```python
from build123d import *

# Parameters (mm, degrees)
SKETCH_1_W                = 100
SKETCH_1_H                = 130
EXTRUDE_1_DEPTH           = 3
SKETCH_2_R                = 2.1
CUT_EXTRUDE_1_DEPTH       = 83.060952956
SKETCH_5_W                = 100
SKETCH_5_H                = 130
EXTRUDE_2_DEPTH           = 3
CUT_EXTRUDE_4_DEPTH       = 164.505351594
CUT_EXTRUDE_4_DEPTH_BACK  = 164.505351594
SKETCH_6_R                = 2.1
CUT_EXTRUDE_5_DEPTH       = 164.505351594
CUT_EXTRUDE_5_DEPTH_BACK  = 164.505351594
SKETCH_7_R                = 2.55
CUT_EXTRUDE_6_DEPTH       = 164.505351594
CUT_EXTRUDE_6_DEPTH_BACK  = 164.505351594
CUT_EXTRUDE_7_DEPTH       = 164.505351594
CUT_EXTRUDE_7_DEPTH_BACK  = 164.505351594
SKETCH_12_W               = 20
SKETCH_12_H               = 20
CUT_EXTRUDE_8_DEPTH       = 164.505351594
CUT_EXTRUDE_8_DEPTH_BACK  = 164.505351594
SKETCH_13_W               = 200
SKETCH_13_H               = 20
CUT_EXTRUDE_9_DEPTH       = 164.505351594
CUT_EXTRUDE_9_DEPTH_BACK  = 164.505351594
SKETCH_14_W               = 5
SKETCH_14_H               = 90
CUT_EXTRUDE_10_DEPTH      = 159.930802553
CUT_EXTRUDE_10_DEPTH_BACK = 159.930802553
SKETCH_15_R               = 1.25
SKETCH_15_R_2             = 22
CUT_EXTRUDE_11_DEPTH      = 159.930802553
CUT_EXTRUDE_11_DEPTH_BACK = 159.930802553
FILLET_1_R                = 1


with BuildPart() as part:
    # 草图1 → 凸台-拉伸1 (new body)
    with BuildSketch(Plane.XY):
        Rectangle(SKETCH_1_W, SKETCH_1_H)
    extrude(amount=EXTRUDE_1_DEPTH)

    # 草图2 → 切除-拉伸1 (cut, through all)
    with BuildSketch(Plane.XY.offset(3)):
        with Locations((-40, 55)):
            Circle(SKETCH_2_R)
        with Locations((-20, 55)):
            Circle(SKETCH_2_R)
        with Locations((0, 55)):
            Circle(SKETCH_2_R)
        with Locations((20, 55)):
            Circle(SKETCH_2_R)
        with Locations((40, 55)):
            Circle(SKETCH_2_R)
        with Locations((-40, -55)):
            Circle(SKETCH_2_R)
        with Locations(Location((40, -55, 0), (0, 0, 180))):
            Circle(SKETCH_2_R)
        with Locations(Location((20, -55, 0), (0, 0, 180))):
            Circle(SKETCH_2_R)
        with Locations(Location((0, -55, 0), (0, 0, 180))):
            Circle(SKETCH_2_R)
        with Locations(Location((-20, -55, 0), (0, 0, 180))):
            Circle(SKETCH_2_R)
    extrude(amount=-CUT_EXTRUDE_1_DEPTH, mode=Mode.SUBTRACT)

    # 草图5 → 凸台-拉伸2 (add)
    with BuildSketch(Plane.XY.offset(3)):
        with Locations((100, 0)):
            Rectangle(SKETCH_5_W, SKETCH_5_H)
    extrude(amount=-EXTRUDE_2_DEPTH)

    # 草图6 → 切除-拉伸4 (cut, two sides: drawn at the far end of the back side and taken through both)
    with BuildSketch(Plane.XY.offset(3).offset(-CUT_EXTRUDE_4_DEPTH_BACK)):
        with Locations((55, 55)):
            Circle(SKETCH_6_R)
        with Locations((70, 55)):
            Circle(SKETCH_6_R)
        with Locations((85, 55)):
            Circle(SKETCH_6_R)
        with Locations((100, 55)):
            Circle(SKETCH_6_R)
        with Locations((115, 55)):
            Circle(SKETCH_6_R)
        with Locations((130, 55)):
            Circle(SKETCH_6_R)
        with Locations((145, 55)):
            Circle(SKETCH_6_R)
        with Locations((145, -55)):
            Circle(SKETCH_6_R)
        with Locations((130, -55)):
            Circle(SKETCH_6_R)
        with Locations((115, -55)):
            Circle(SKETCH_6_R)
        with Locations((100, -55)):
            Circle(SKETCH_6_R)
        with Locations((85, -55)):
            Circle(SKETCH_6_R)
        with Locations((70, -55)):
            Circle(SKETCH_6_R)
        with Locations((55, -55)):
            Circle(SKETCH_6_R)
    extrude(amount=CUT_EXTRUDE_4_DEPTH + CUT_EXTRUDE_4_DEPTH_BACK, mode=Mode.SUBTRACT)

    # 草图7 → 切除-拉伸5 (cut, two sides: drawn at the far end of the back side and taken through both)
    with BuildSketch(Plane(origin=(0, 0, 0), x_dir=(-1, 0, 0), z_dir=(0, 0, -1)).offset(-CUT_EXTRUDE_5_DEPTH_BACK)):
        with Locations((-140, -30)):
            Circle(SKETCH_7_R)
        with Locations((-120, -30)):
            Circle(SKETCH_7_R)
        with Locations((-100, -30)):
            Circle(SKETCH_7_R)
        with Locations((-80, -30)):
            Circle(SKETCH_7_R)
        with Locations((-60, -30)):
            Circle(SKETCH_7_R)
        with Locations((-40, -30)):
            Circle(SKETCH_7_R)
        with Locations((-20, -30)):
            Circle(SKETCH_7_R)
        with Locations((0, -30)):
            Circle(SKETCH_7_R)
        with Locations((20, -30)):
            Circle(SKETCH_7_R)
        with Locations((40, -30)):
            Circle(SKETCH_7_R)
    extrude(amount=CUT_EXTRUDE_5_DEPTH + CUT_EXTRUDE_5_DEPTH_BACK, mode=Mode.SUBTRACT)

    # 草图11 → 切除-拉伸6 (cut, two sides: drawn at the far end of the back side and taken through both)
    with BuildSketch(Plane.XY.offset(3).offset(-CUT_EXTRUDE_6_DEPTH_BACK)):
        with BuildLine():
            Line((74.5, 19.5), (74.5, 65))
            Line((74.5, 65), (25.5, 65))
            Line((25.5, 65), (25.5, 19.5))
            ThreePointArc((25.5, 19.5), (50, -5), (74.5, 19.5))
        make_face()
    extrude(amount=CUT_EXTRUDE_6_DEPTH + CUT_EXTRUDE_6_DEPTH_BACK, mode=Mode.SUBTRACT)

    # 草图12 → 切除-拉伸7 (cut, two sides: drawn at the far end of the back side and taken through both)
    with BuildSketch(Plane.XY.offset(3).offset(-CUT_EXTRUDE_7_DEPTH_BACK)):
        with Locations((-40, 55)):
            Rectangle(SKETCH_12_W, SKETCH_12_H)
        with Locations((140, 55)):
            Rectangle(SKETCH_12_W, SKETCH_12_H)
    extrude(amount=CUT_EXTRUDE_7_DEPTH + CUT_EXTRUDE_7_DEPTH_BACK, mode=Mode.SUBTRACT)

    # 草图13 → 切除-拉伸8 (cut, two sides: drawn at the far end of the back side and taken through both)
    with BuildSketch(Plane.XY.offset(3).offset(-CUT_EXTRUDE_8_DEPTH_BACK)):
        with Locations((50, -55)):
            Rectangle(SKETCH_13_W, SKETCH_13_H)
    extrude(amount=CUT_EXTRUDE_8_DEPTH + CUT_EXTRUDE_8_DEPTH_BACK, mode=Mode.SUBTRACT)

    # 草图14 → 切除-拉伸9 (cut, two sides: drawn at the far end of the back side and taken through both)
    with BuildSketch(Plane.XY.offset(3).offset(-CUT_EXTRUDE_9_DEPTH_BACK)):
        with Locations((147.5, 0)):
            Rectangle(SKETCH_14_W, SKETCH_14_H)
    extrude(amount=CUT_EXTRUDE_9_DEPTH + CUT_EXTRUDE_9_DEPTH_BACK, mode=Mode.SUBTRACT)

    # 草图15 → 切除-拉伸10 (cut, two sides: drawn at the far end of the back side and taken through both)
    with BuildSketch(Plane(origin=(0, 0, 0), x_dir=(-1, 0, 0), z_dir=(0, 0, -1)).offset(-CUT_EXTRUDE_10_DEPTH_BACK)):
        with Locations((10.74, 4.505)):
            Circle(SKETCH_15_R)
        with Locations((31.96195252, -32.2525)):
            Circle(SKETCH_15_R)
        with Locations((-10.48195252, -32.2525)):
            Circle(SKETCH_15_R)
        with Locations((10.74, -20)):
            Circle(SKETCH_15_R_2)
    extrude(amount=CUT_EXTRUDE_10_DEPTH + CUT_EXTRUDE_10_DEPTH_BACK, mode=Mode.SUBTRACT)

    # 草图16 → 切除-拉伸11 (cut, two sides: drawn at the far end of the back side and taken through both)
    with BuildSketch(Plane.XY.offset(3).offset(-CUT_EXTRUDE_11_DEPTH_BACK)):
        Polygon((6, 10.5), (6, 28.5), (25.5, 28.5), (74.5, 28.5), (123, 28.5), (123, 10.5), (74.5, 10.5), (25.5, 10.5), align=None)
    extrude(amount=CUT_EXTRUDE_11_DEPTH + CUT_EXTRUDE_11_DEPTH_BACK, mode=Mode.SUBTRACT)

    # 圆角1
    fillet_1_edges = [part.edges().sort_by_distance(p)[0] for p in [
        (74.5, 28.5, 1.5),
        (27.21294227, 10.5, 1.5),
        (72.78705773, 10.5, 1.5),
        (123, 10.5, 1.5),
        (25.5, 28.5, 1.5),
        (6, 28.5, 1.5),
        (6, 10.5, 1.5),
        (123, 28.5, 1.5),
    ]]
    fillet(fillet_1_edges, radius=FILLET_1_R)


solid = part.part
```
Here's how the part is built. I have some questions about the finished solid (model axes, mm). Coordinates: 2 decimals unless noted, no trailing zeros. Loops run counter-clockwise (first coordinate to the right, second up) from the corner with the lowest first, then second, coordinate; pieces in that order, holes last. Notation, with made-up numbers: M 79.25,56 L 122.25,56 A3 cw 122.25,60 Z; hole C 10.25,33.5 d4. An arc over 180 degrees is marked long. One line per item, written item: value.
1. Will these pins go through, and if not, where does the flat tip stop? pin 1 Ø1.5 at (y, z) = (62, 1) entering from +X; pin 2 Ø4 at (x, y) = (100, 55) entering from -Z; pin 3 Ø1.5 at (x, z) = (137.5, 1.5) entering from +Y; pin 4 Ø6.5 at (x, y) = (40, -30) entering from -Z.
Geometry says:
pin 1: stops at x = 130
pin 2: passes through
pin 3: stops at y = 45
pin 4: stops at z = 0
2. Please list where these lines run through material, in increasing order: probe 1 along Y at (x, z) = (20, 1.8); probe 2 along Y at (x, z) = (85.5, 1.6); probe 3 along X at (y, z) = (22.5, 2.85).
Geometry says:
probe 1: y = -45 to -32.55, -27.45 to 10.5, 28.5 to 52.9, 57.1 to 65
probe 2: y = -45 to 10.5, 28.5 to 52.96, 57.04 to 65
probe 3: x = -50 to 6, 123 to 145
3. Thinking about a two-plate mould opening in X: for faces 1 (the cylindrical face through (50, -5, 1)), 2 (the flat face through (46, -14, 0)), 3 (the cylindrical face through (62.548, -29.888, 1.521)), which applies, +X half, -X half, draft (parallel to the pull), parting line (faces both ways), or undercut?
Geometry says:
face 1: undercut
face 2: draft
face 3: undercut
4. Imagine slicing it at A-A (x = 100). List the corners of the cut face in (y, z) for me, and give its area (3 significant figures).
Geometry says:
outline: M -45,0 L -32.55,0 L -32.55,3 L -45,3 Z; M -27.45,0 L 10.5,0 L 10.5,3 L -27.45,3 Z; M 28.5,0 L 52.9,0 L 52.9,3 L 28.5,3 Z; M 57.1,0 L 65,0 L 65,3 L 57.1,3 Z
area: 248 mm2
5. Imagine slicing it at B-B (y = 17.5). List the corners of the cut face in (x, z) for me, and give its area (3 significant figures).
Geometry says:
outline: M -50,0 L 6,0 L 6,3 L -50,3 Z; M 123,0 L 145,0 L 145,3 L 123,3 Z
area: 234 mm2
6. Imagine slicing it at C-C (x = 40). List the corners of the cut face in (y, z) for me, and give its area (3 significant figures).
Geometry says:
outline: M -45,0 L -32.55,0 L -32.55,3 L -45,3 Z; M -27.45,0 L -2.87,0 L -2.87,3 L -27.45,3 Z
area: 111 mm2
7. Imagine slicing it at D-D (x = -20). List the corners of the cut face in (y, z) for me.
Geometry says:
outline: M -45,0 L -39.96,0 L -39.96,3 L -45,3 Z; M -0.04,0 L 52.9,0 L 52.9,3 L -0.04,3 Z; M 57.1,0 L 65,0 L 65,3 L 57.1,3 Z
